Print and shaded views of the part. All mm, measured from the part's lowest x, y and z. A direction names the side the tool comes from. Give positions to 0.01 mm unless a question says otherwise; leave off trailing zeros. Loops run counter-clockwise (first coordinate to the right, second up) from the corner with the lowest first, then second, coordinate; pieces in that order, holes last. Notation, with made-up numbers: M -9.75,63.25 L 30.25,63.25 A19 ccw 30.25,89.25 Z; hole C 66,16.5 d10. An arc over 180 degrees is marked long. Answer in a Markdown table with one row per item.
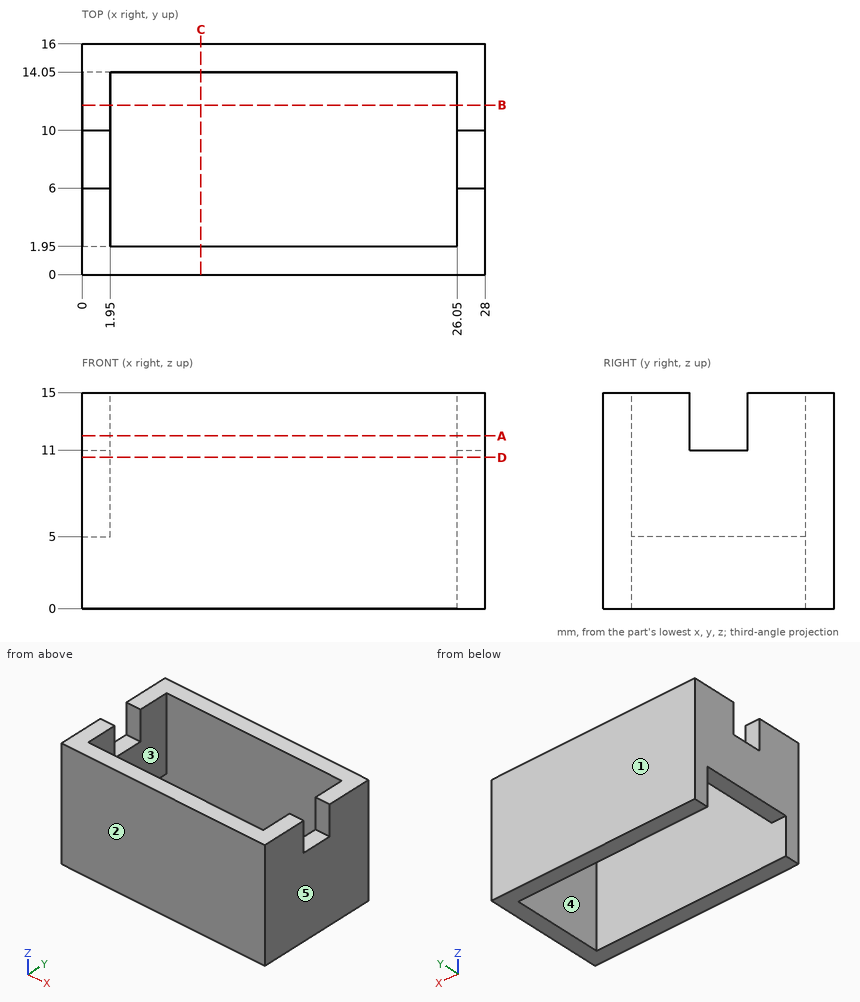
(1) Saw through at D-D, the plane z = 10.5. Give the cut face in (x, y), and give its area (3 significant figures).
Established:
| item | result |
|---|---|
| outline | M 0,0 L 28,0 L 28,16 L 0,16 Z; hole M 1.95,1.95 L 26.05,1.95 L 26.05,14.05 L 1.95,14.05 Z |
| area | 156 mm2 |
(2) Wall check: L1, parallel to X at y = 2.5, z = 11; L2, parallel to Y at x = 2.75, z = 2.75. Give the ranges that are in metal, low to high.
Established:
| item | result |
|---|---|
| L1 | x = 0 to 1.95, 26.05 to 28 |
| L2 | y = 0 to 1.95, 14.05 to 16 |
(3) Which spindle directions (+Z, -Z, +X, -X, +Y, -Y) get a long thin tool onto all of the face, cutting with end or side? Do the marked faces 4 and 5. Say none if no direction does.
Established:
| item | result |
|---|---|
| face 4 | +Z, -Z |
| face 5 | +Z, -Z, +X, +Y, -Y |
(4) Saw through at A-A, the plane z = 12. Give the cut face in (x, y), and give its area (3 significant figures).
Established:
| item | result |
|---|---|
| outline | M 0,0 L 28,0 L 28,6 L 26.05,6 L 26.05,1.95 L 1.95,1.95 L 1.95,6 L 0,6 Z; M 0,10 L 1.95,10 L 1.95,14.05 L 26.05,14.05 L 26.05,10 L 28,10 L 28,16 L 0,16 Z |
| area | 141 mm2 |
(5) Saw through at B-B, the plane y = 11.75. Give the cut face in (x, z).
Established:
| item | result |
|---|---|
| outline | M 0,5 L 1.95,5 L 1.95,15 L 0,15 Z; M 26.05,0 L 28,0 L 28,15 L 26.05,15 Z |
(6) Flat gauge pins, fed straight in: P1, Ø1, axis at x = 0.5, z = 12.5, coming from the -Y side; P2, Ø1, axis at x = 1, y = 7.5, coming from the +Z side; P3, Ø1.6, axis at x = 0.5, y = 10, coming from the -Z side. Where does each tip first touch, or does it go through?
Established:
| item | result |
|---|---|
| P1 | stops at y = 0 |
| P2 | stops at z = 11 |
| P3 | stops at z = 5 |
(7) Saw through at C-C, the plane x = 8.25. Give the cut face in (y, z).
Established:
| item | result |
|---|---|
| outline | M 0,0 L 1.95,0 L 1.95,15 L 0,15 Z; M 14.05,0 L 16,0 L 16,15 L 14.05,15 Z |
(8) Mould opens along Y. For the marked faces 1, 2 and 3 say: pulls with the +Y half, pulls with the -Y half, needs draft (parallel to the pull), parting line crosses it, or undercut.
Established:
| item | result |
|---|---|
| face 1 | pulls with the +Y half |
| face 2 | pulls with the -Y half |
| face 3 | undercut |
